Could you check a few things on this model? Use its own coordinates, in mm. Face numbers are marked on the shaded views. A direction names the side the tool comes from. Give positions to 0.01 mm unless a question says otherwise; leave off trailing zeros. One line per item, written item: value.
```python
from build123d import *
from build123d.topology import SkipClean

# Parameters (mm, degrees)
SKETCH_1_R          = 20
SKETCH_1_R_2        = 4.55
EXTRUDE_1_DEPTH     = 3
SKETCH_4_R          = 1.25
CUT_EXTRUDE_3_DEPTH = 11
SKETCH_5_R          = 1.25
CUT_EXTRUDE_4_DEPTH = 1
SKETCH_7_R          = 20
SKETCH_7_R_2        = 9.5
EXTRUDE_2_DEPTH     = 1
EXTRUDE_START       = 0.2
SKETCH_9_R          = 20
SKETCH_9_R_2        = 9.5
EXTRUDE_3_DEPTH     = 0.2
SKETCH_10_R         = 19.25
SKETCH_10_R_2       = 17.25
CUT_EXTRUDE_6_DEPTH = 1
FILLET_1_R          = 1
SKETCH_11_R         = 20
CUT_EXTRUDE_7_DEPTH = 0.2
SKETCH_13_R         = 1.65
CUT_EXTRUDE_8_DEPTH = 29.565713714


with BuildPart() as part:
    # 草图1 → 凸台-拉伸1 (new body)
    with BuildSketch(Plane.XY):
        Circle(SKETCH_1_R)
        Circle(SKETCH_1_R_2, mode=Mode.SUBTRACT)
    extrude(amount=EXTRUDE_1_DEPTH)

    # 草图4 → 切除-拉伸3 (cut)
    with BuildSketch(Plane.XY.offset(3)):
        with Locations((0, 7.25)):
            Circle(SKETCH_4_R)
        with Locations((7.25, 0)):
            Circle(SKETCH_4_R)
        with Locations((0, -7.25)):
            Circle(SKETCH_4_R)
        with Locations((-7.25, 0)):
            Circle(SKETCH_4_R)
    extrude(amount=-CUT_EXTRUDE_3_DEPTH, mode=Mode.SUBTRACT)

    # 草图5 → 切除-拉伸4 (cut)
    with BuildSketch(Plane.XY.offset(3)):
        with BuildLine():
            ThreePointArc((-5.382359347, 2.08612521), (-10.05, 0), (-5.382359347, -2.08612521))
            ThreePointArc((-5.382359347, -2.08612521), (-4.565967837, -1.842389611), (-3.858009404, -2.316411759))
            ThreePointArc((-3.858009404, -2.316411759), (-3.181980515, -3.181980515), (-2.316411759, -3.858009404))
            ThreePointArc((-2.316411759, -3.858009404), (-1.842389611, -4.565967837), (-2.08612521, -5.382359347))
            ThreePointArc((-2.08612521, -5.382359347), (0, -10.05), (2.08612521, -5.382359347))
            ThreePointArc((2.08612521, -5.382359347), (1.842389611, -4.565967837), (2.316411759, -3.858009404))
            ThreePointArc((2.316411759, -3.858009404), (3.181980515, -3.181980515), (3.858009404, -2.316411759))
            ThreePointArc((3.858009404, -2.316411759), (4.565967837, -1.842389611), (5.382359347, -2.08612521))
            ThreePointArc((5.382359347, -2.08612521), (10.05, 0), (5.382359347, 2.08612521))
            ThreePointArc((5.382359347, 2.08612521), (4.565967837, 1.842389611), (3.858009404, 2.316411759))
            ThreePointArc((3.858009404, 2.316411759), (3.181980515, 3.181980515), (2.316411759, 3.858009404))
            ThreePointArc((2.316411759, 3.858009404), (1.842389611, 4.565967837), (2.08612521, 5.382359347))
            ThreePointArc((2.08612521, 5.382359347), (0, 10.05), (-2.08612521, 5.382359347))
            ThreePointArc((-2.08612521, 5.382359347), (-1.842389611, 4.565967837), (-2.316411759, 3.858009404))
            ThreePointArc((-2.316411759, 3.858009404), (-3.181980515, 3.181980515), (-3.858009404, 2.316411759))
            ThreePointArc((-3.858009404, 2.316411759), (-4.565967837, 1.842389611), (-5.382359347, 2.08612521))
        make_face()
        with Locations((0, -7.25)):
            Circle(SKETCH_5_R, mode=Mode.SUBTRACT)
        with Locations((-7.25, 0)):
            Circle(SKETCH_5_R, mode=Mode.SUBTRACT)
        with Locations((7.25, 0)):
            Circle(SKETCH_5_R, mode=Mode.SUBTRACT)
        with Locations((0, 7.25)):
            Circle(SKETCH_5_R, mode=Mode.SUBTRACT)
    extrude(amount=-CUT_EXTRUDE_4_DEPTH, mode=Mode.SUBTRACT)

    # 草图7 → 凸台-拉伸2 (add, symmetric)
    with SkipClean():  # the faces are left unmerged after this step: merging them gives an invalid solid
        with BuildSketch(Plane(origin=(0, 0, 0), x_dir=(-1, 0, 0), z_dir=(0, 0, -1))):
            Circle(SKETCH_7_R)
            with Locations(Location((0, 0, 0), (0, 0, 180))):
                Circle(SKETCH_7_R_2, mode=Mode.SUBTRACT)
        extrude(amount=EXTRUDE_2_DEPTH, both=True)

    # 草图9 → 凸台-拉伸3 (add)
    with BuildSketch(Plane(origin=(0, 0, -1), x_dir=(-1, 0, 0), z_dir=(0, 0, -1)).offset(EXTRUDE_START)):
        Circle(SKETCH_9_R)
        with Locations(Location((0, 0, 0), (0, 0, 180))):
            Circle(SKETCH_9_R_2, mode=Mode.SUBTRACT)
    extrude(amount=-EXTRUDE_3_DEPTH)

    # 草图10 → 切除-拉伸6 (cut)
    with BuildSketch(Plane(origin=(0, 0, -1.2), x_dir=(-1, 0, 0), z_dir=(0, 0, -1))):
        Circle(SKETCH_10_R)
        Circle(SKETCH_10_R_2, mode=Mode.SUBTRACT)
    extrude(amount=-CUT_EXTRUDE_6_DEPTH, mode=Mode.SUBTRACT)

    # 圆角1
    fillet_1_edges = [part.edges().sort_by_distance(p)[0] for p in [
        (19.25, 0, -0.2),
        (17.25, 0, -0.2),
    ]]
    fillet(fillet_1_edges, radius=FILLET_1_R - 0.0001)  # a hair under: the kernel refuses the full size

    # 草图11 → 切除-拉伸7 (cut)
    with BuildSketch(Plane(origin=(0, 0, -1.2), x_dir=(-1, 0, 0), z_dir=(0, 0, -1))):
        Circle(SKETCH_11_R)
    extrude(amount=-CUT_EXTRUDE_7_DEPTH, mode=Mode.SUBTRACT)

    # 草图13 → 切除-拉伸8 (cut, through all)
    with BuildSketch(Plane(origin=(0, 0, -1), x_dir=(-1, 0, 0), z_dir=(0, 0, -1))):
        with Locations((0, 15)):
            Circle(SKETCH_13_R)
        with Locations((12.990381057, -7.5)):
            Circle(SKETCH_13_R)
        with Locations((-12.990381057, -7.5)):
            Circle(SKETCH_13_R)
    extrude(amount=-CUT_EXTRUDE_8_DEPTH, mode=Mode.SUBTRACT)


solid = part.part
```
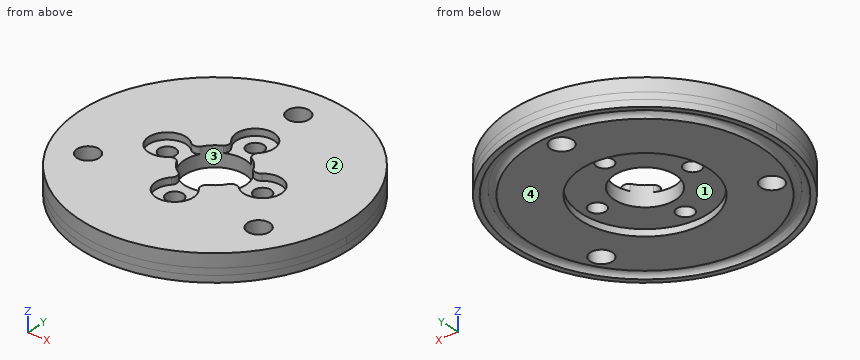
1) Suppose I cut it at A-A, the plane x = 0. State how many separate pieces and enclosed holes the cut face has, then the cut area to 3 significant figures.
Answer below:
separate pieces: 5
enclosed holes: 0
area: 77.2 mm2
2) If I drill on line 1 along X through (y, z) = (-0.5, 1.9); line 2 along Y through (x, z) = (0.5, 2.1) (3 decimals); line 3 along X through (y, z) = (-8.5, -0.35), over which ranges is the centre line in solid material (lowest first)?
Answer below:
line 1: x = -19.99 to -8.4, -6.1 to -4.52, 4.52 to 6.1, 8.4 to 19.99
line 2: y = -19.994 to -10.005, 10.005 to 13.428, 16.572 to 19.994
line 3: x = -18.1 to -16.74, -15.55 to -14.3, -11.68 to -4.24, 4.24 to 11.68, 14.3 to 15.55, 16.74 to 18.1
3) We'd pull the mould along Y, two halves only. Please class the marked faces 3 and 4: +Y half, -Y half, draft (parallel to the pull), parting line (faces both ways), or undercut.
Answer below:
face 3: undercut
face 4: draft
4) For P1, Ø5, axis at x = 7.25, y = 0, coming from the +Z side; P2, Ø4, axis at x = -12.99, y = -7.5, coming from the -Z side; P3, Ø4, axis at x = 7.25, y = 0, coming from the -Z side; P4, Ø2, axis at x = 0, y = 15, coming from the -Z side, each with a flat end and sliding along its axis, tell me the tip position at first contact or that it passes through.
Answer below:
P1: stops at z = 2
P2: stops at z = -1
P3: stops at z = 0
P4: passes through
5) For the marked faces 1 and 2, which set-ups out of +Z, -Z, +X, -X, +Y, -Y let a thin tool reach every point of the face, with its end or its side?
Answer below:
face 1: -Z
face 2: +Z, +X, -X, +Y, -Y
